Part print with two shaded views. Sizes in mm from the minimum x, y, z corner. A direction names the side the tool comes from. Round coordinates to 2 decimals unless told otherwise and drop trailing zeros. Loops run counter-clockwise (first coordinate to the right, second up) from the corner with the lowest first, then second, coordinate; pieces in that order, holes last. Notation, with made-up numbers: (9.5, 32.25) - (46.5, 32.25) arc R25 ccw to (46.5, 64.25) - close; hole circle Ø2 at (74.5, 55). An arc over 180 degrees is marked (long way). Use a Markdown table: item, result.
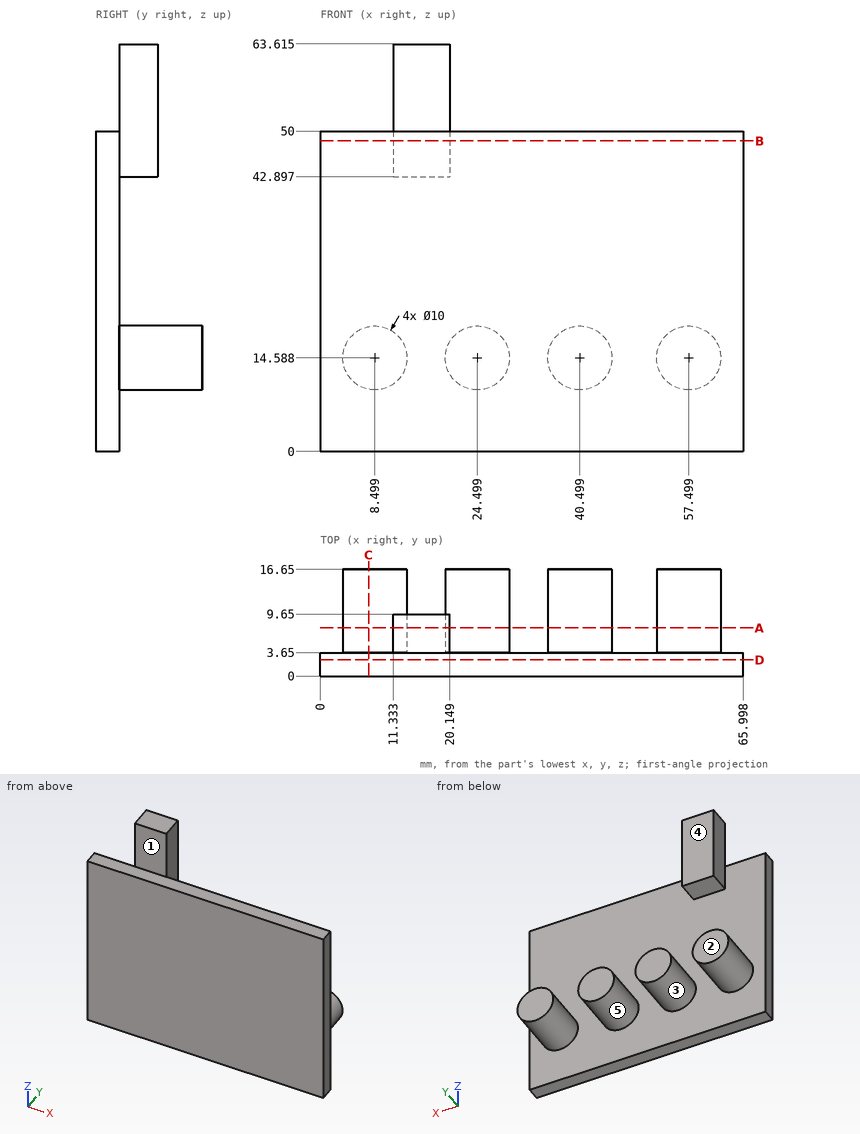
Q1. Probe line 1 (X direction, y = 6.75, z = 12) (1 decimal); line 2 (Y direction, x = 27, z = 40.5); line 3 (Y direction, x = 18, z = 44.5). List the from-to ranges inside material, lowest first.
Results found:
| item | result |
|---|---|
| line 1 | x = 4.2 to 12.8, 20.2 to 28.8, 36.2 to 44.8, 53.2 to 61.8 |
| line 2 | y = 0 to 3.65 |
| line 3 | y = 0 to 9.65 |
Q2. Cut at A-A, the plane y = 7.5. Count the separate pieces of the cut face and the enclosed holes in it, plus the area to 3 significant figures.
Results found:
| item | result |
|---|---|
| separate pieces | 5 |
| enclosed holes | 0 |
| area | 497 mm2 |
Q3. Which spindle directions (+Z, -Z, +X, -X, +Y, -Y) get a long thin tool onto all of the face, cutting with end or side? Do the marked faces 1, 2 and 3. Say none if no direction does.
Results found:
| item | result |
|---|---|
| face 1 | +Z, +X, -X, -Y |
| face 2 | +Z, -Z, +X, -X, +Y |
| face 3 | +Y |
Q4. Drop flat-ended pins along their axis: pin 1 (7 mm diameter, centred on x = 15, z = 56, fed in from -Y); pin 2 (4 mm diameter, centred on x = 27, y = 1.5, fed in from +Z); pin 3 (3 mm diameter, centred on y = 7, z = 41, fed in from -X) (1 decimal); pin 4 (4 mm diameter, centred on y = 3.5, z = 8, fed in from -X). Give the stop position or say it passes through.
Results found:
| item | result |
|---|---|
| pin 1 | stops at y = 3.65 |
| pin 2 | stops at z = 50 |
| pin 3 | passes through |
| pin 4 | stops at x = 0 |
Q5. Pull direction X, two halves, no side cores. Call the marked faces 4 and 5: pulls with the +X half, pulls with the -X half, needs draft (parallel to the pull), parting line crosses it, or undercut.
Results found:
| item | result |
|---|---|
| face 4 | needs draft |
| face 5 | undercut |
Q6. Cut at B-B, the plane z = 48.5. List the corners of the cut face in (x, y), plus the area to 3 significant figures.
Results found:
| item | result |
|---|---|
| outline | (0, 0) - (66, 0) - (66, 3.65) - (20.15, 3.65) - (20.15, 9.65) - (11.33, 9.65) - (11.33, 3.65) - (0, 3.65) - close |
| area | 294 mm2 |
Q7. Cut at C-C, the plane x = 7.5. List the corners of the cut face in (y, z).
Results found:
| item | result |
|---|---|
| outline | (0, 0) - (3.65, 0) - (3.65, 9.69) - (16.65, 9.69) - (16.65, 19.49) - (3.65, 19.49) - (3.65, 50) - (0, 50) - close |
Q8. Cut at D-D, the plane y = 2.5. List the corners of the cut face in (x, z), plus the area to 3 significant figures.
Results found:
| item | result |
|---|---|
| outline | (0, 0) - (66, 0) - (66, 50) - (0, 50) - close |
| area | 3,300 mm2 |
